Geometry: see drawing. Coordinates: mm, zero at the bounding-box minimum. Coordinates: 2 decimals unless noted, no trailing zeros. Order: outer loops, then holes, each group sorted by start corner. A loop starts at its lowest first (then second) coordinate and runs counter-clockwise, first axis right, second up. Notation, with made-up numbers: M 29,47.25 L 53,47.25 A21 ccw 53,65.25 Z; hole C 4,-11.5 d5. An arc over 180 degrees is marked long. Answer in a Markdown table with one row per item.
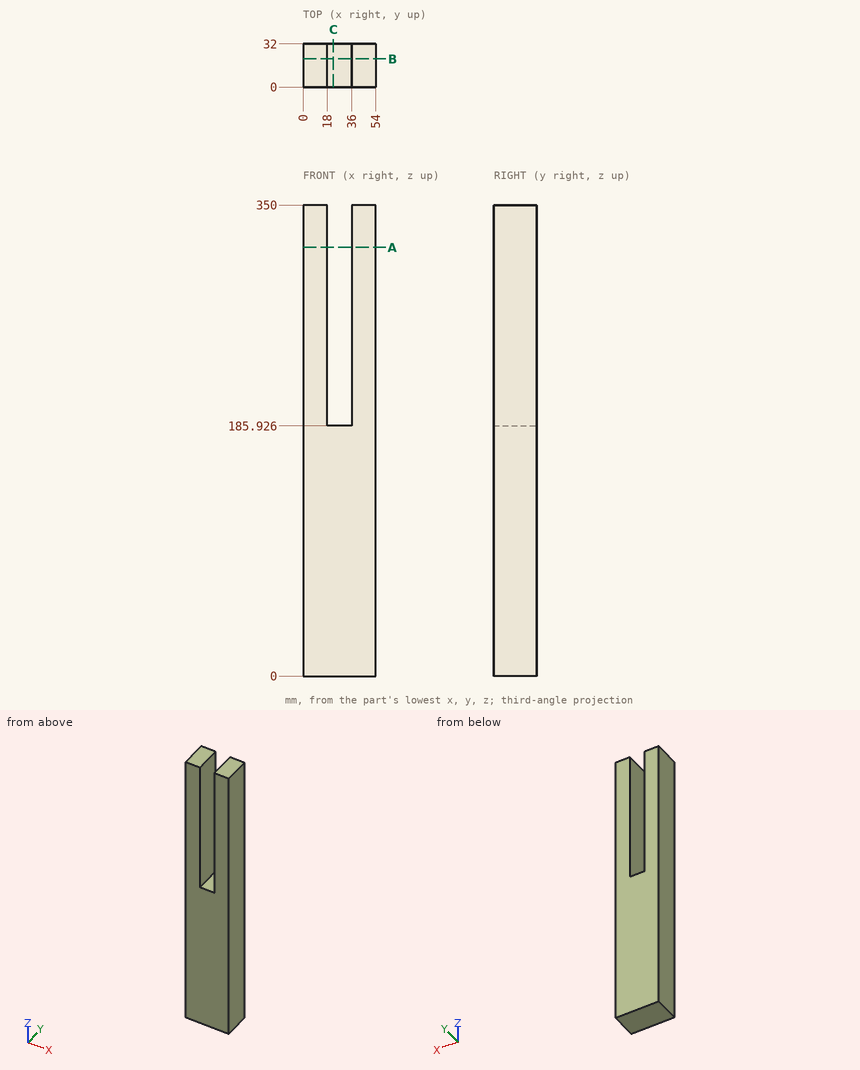
1) Cut plane B-B, the plane y = 21. Output: boundary loops of the cut face in (x, z), and give its area (3 significant figures).
Resolved:
| item | result |
|---|---|
| outline | M 0,0 L 54,0 L 54,350 L 36,350 L 36,185.93 L 18,185.93 L 18,350 L 0,350 Z |
| area | 15,900 mm2 |
2) Material intervals for probe 1 along X at (y, z) = (30, 290); probe 2 along Z at (x, y) = (28.5, 16.5), sorted ascending.
Resolved:
| item | result |
|---|---|
| probe 1 | x = 0 to 18, 36 to 54 |
| probe 2 | z = 0 to 185.93 |
3) Cut plane A-A, the plane z = 318.5. Output: boundary loops of the cut face in (x, y), and give its area (3 significant figures).
Resolved:
| item | result |
|---|---|
| outline | M 0,0 L 18,0 L 18,32 L 0,32 Z; M 36,0 L 54,0 L 54,32 L 36,32 Z |
| area | 1,150 mm2 |
4) Cut plane C-C, the plane x = 22.5. Output: boundary loops of the cut face in (y, z).
Resolved:
| item | result |
|---|---|
| outline | M 0,0 L 32,0 L 32,185.93 L 0,185.93 Z |
5) Contact query for flat-ended pins moving along their axis: pin 1 (5 mm diameter, centred on x = 30.5, y = 22, fed in from +Z); pin 2 (4 mm diameter, centred on x = 38.5, z = 245.5, fed in from -Y). Output: stop coordinate, or through.
Resolved:
| item | result |
|---|---|
| pin 1 | stops at z = 185.93 |
| pin 2 | stops at y = 0 |
